The drawing under review shows one solid part. Ordinate dimensions are in mm from its lowest x, y, z. A direction names the side the tool comes from. Give positions to 0.01 mm unless a question says otherwise; leave off trailing zeros. Order: outer loops, then holes, each group sorted by start corner. A loop starts at its lowest first (then second) coordinate and runs counter-clockwise, first axis right, second up. Notation, with made-up numbers: (76, 38.25) -> (99, 38.25) arc R23 cw to (99, 46.25) -> close; hole circle Ø5 at (62, 18). An arc over 180 degrees is marked (long way). Return JSON: item names as keys, results as strings. Group by question number.
1) Insertion check: P1, Ø4.5, axis at y = 5.75, z = 36.75, coming from the +X side; P2, Ø1, axis at x = 42, y = 62.5, coming from the -Z side; P3, Ø1, axis at y = 12, z = 26.5, coming from the -X side; P4, Ø0.6, axis at y = 62.5, z = 36.5, coming from the -X side. Each pin has a flat end and moves straight along its axis. Give the tip position at first contact, or say it passes through.
2) To check wall thickness, follow line 1 along Z through (x, y) = (58.85, 36.75); line 2 along Z through (x, y) = (22.5, 10.5); line 3 along X through (y, z) = (31.5, 5). State the ranges of each line that lie inside material, in increasing order.
3) Add section B-B (z = 5.75). Give the boundary of the cut face in (x, y), then the cut area to 3 significant figures.
4) For the marked faces 4, 5 and 6, list the 3-axis set-ups (+Z, -Z, +X, -X, +Y, -Y) from which the entire face can be reached by the end or side of a thin tool; tool diameter is ignored.
5) Add section C-C (z = 36.75). Give the boundary of the cut face in (x, y), then the cut area to 3 significant figures.
6) The part is to be moulded in two halves that separate along Y. For the marked faces 1, 2 and 3, say which applies: released by +Y, released by -Y, zero draft, split by the parting line, or undercut.
7) Add section D-D (z = 21.25). Give the boundary of the cut face in (x, y).
8) Add section A-A (y = 36.75). Give the boundary of the cut face in (x, z), then the cut area to 3 significant figures.
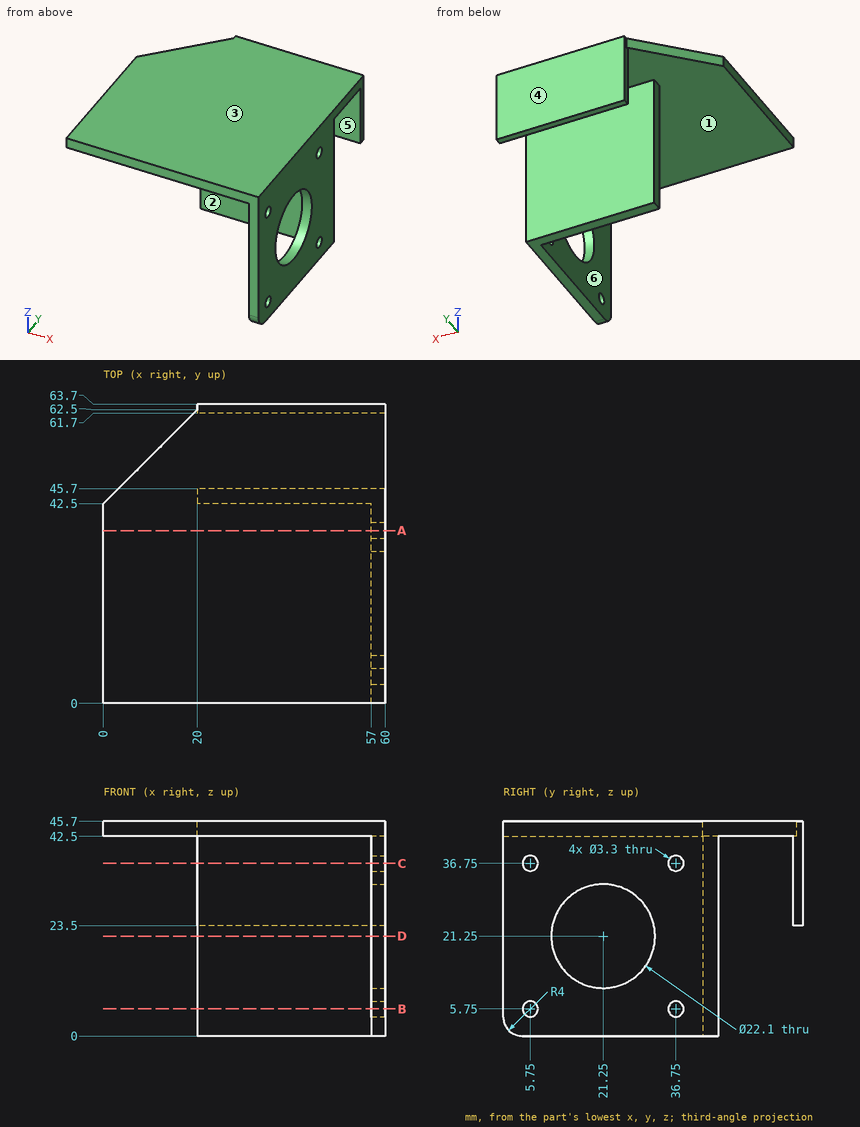
Evaluation:
{
 "1": {"P1": "x = 60", "P2": "z = 23.5", "P3": "x = 57", "P4": "x = 20"},
 "2": {"line 1": "0 to 4.1, 7.4 to 35.1, 38.4 to 45.7", "line 2": "42.5 to 45.7", "line 3": "57 to 60"},
 "3": {"outline": "(20, 42.5) -> (57, 42.5) -> (57, 38.4) -> (60, 38.4) -> (60, 45.7) -> (20, 45.7) -> close; (57, 0) -> (60, 0) -> (60, 4.1) -> (57, 4.1) -> close; (57, 7.4) -> (60, 7.4) -> (60, 35.1) -> (57, 35.1) -> close", "area": "236 mm^2"},
 "4": {"face 4": "+Z, -Z, +X, -X, +Y", "face 5": "-Z, +X, -X", "face 6": "-Z, -X, -Y"},
 "5": {"outline": "(20, 42.5) -> (57, 42.5) -> (57, 38.4) -> (60, 38.4) -> (60, 45.7) -> (20, 45.7) -> close; (20, 61.7) -> (60, 61.7) -> (60, 63.7) -> (20, 63.7) -> close; (57, 0) -> (60, 0) -> (60, 4.1) -> (57, 4.1) -> close; (57, 7.4) -> (60, 7.4) -> (60, 35.1) -> (57, 35.1) -> close", "area": "316 mm^2"},
 "6": {"face 1": "undercut", "face 2": "released by -Y", "face 3": "zero draft"},
 "7": {"outline": "(20, 42.5) -> (57, 42.5) -> (57, 32.3) -> (60, 32.3) -> (60, 45.7) -> (20, 45.7) -> close; (57, 0) -> (60, 0) -> (60, 10.2) -> (57, 10.2) -> close"},
 "8": {"outline": "(0, 42.5) -> (57, 42.5) -> (57, 38.4) -> (60, 38.4) -> (60, 45.7) -> (0, 45.7) -> close; (57, 0) -> (60, 0) -> (60, 4.1) -> (57, 4.1) -> close; (57, 7.4) -> (60, 7.4) -> (60, 35.1) -> (57, 35.1) -> close", "area": "300 mm^2"}
}
